Input: part model. Units: mm. Frame: model coordinates. A direction names the side the tool comes from. Coordinates: 2 decimals unless noted, no trailing zeros. Loops run counter-clockwise (first coordinate to the right, second up) from the corner with the lowest first, then second, coordinate; pieces in that order, holes last. Notation, with made-up numbers: (6, 2.5) - (26, 2.5) arc R12 cw to (26, 11.5) - close; hole circle Ø6 at (74, 28.25). An arc over 180 degrees is marked (long way). Write item = value, one per line. Start each with the question number.
from build123d import *

# Parameters (mm, degrees)
BOSS_EXTRUDE1_DEPTH = 2.54
SKETCH2_R           = 5.207
BOSS_EXTRUDE2_DEPTH = 12.7
SKETCH6_R           = 4
BOSS_EXTRUDE3_DEPTH = 5.08
FILLET1_R           = 0.508


with BuildPart() as part:
    # Sketch1 → Boss-Extrude1 (new body)
    with BuildSketch(Plane(origin=(0, 0, 0), x_dir=(1, 0, 0), z_dir=(0, 1, 0))):
        Polygon((10.998522628, 0), (5.499261314, 9.525), (-5.499261314, 9.525), (-10.998522628, 0), (-5.499261314, -9.525), (5.499261314, -9.525), align=None)
    extrude(amount=BOSS_EXTRUDE1_DEPTH)

    # Sketch2 → Boss-Extrude2 (add)
    with BuildSketch(Plane(origin=(0, 2.54, 0), x_dir=(1, 0, 0), z_dir=(0, 1, 0))):
        Circle(SKETCH2_R)
    extrude(amount=BOSS_EXTRUDE2_DEPTH)

    # Sketch6 → Boss-Extrude3 (add)
    with BuildSketch(Plane(origin=(0, 0, 0), x_dir=(-1, 0, 0), z_dir=(0, -1, 0))):
        Circle(SKETCH6_R)
    extrude(amount=BOSS_EXTRUDE3_DEPTH)

    # Fillet1
    fillet1_edges = [part.edges().sort_by_distance(p)[0] for p in [
        (0, 2.54, -9.525),
        (5.499261314, 1.27, 9.525),
        (-5.499261314, 1.27, 9.525),
        (-10.998522628, 1.27, 0),
        (-5.499261314, 1.27, -9.525),
        (5.499261314, 1.27, -9.525),
        (10.998522628, 1.27, 0),
        (-8.248891971, 2.54, -4.7625),
        (-8.248891971, 2.54, 4.7625),
        (0, 2.54, 9.525),
        (8.248891971, 2.54, 4.7625),
        (8.248891971, 2.54, -4.7625),
    ]]
    fillet(fillet1_edges, radius=FILLET1_R)


solid = part.part
Item 1: Access query for faces 1 (the flat face through (0, 1, -9.525)), 2 (the flat face through (4, 2.54, -4)), 3 (the cylindrical face through (0.867, -2.504, 3.905)). Directions: +Z, -Z, +X, -X, +Y, -Y. A direction counts if a zero-diameter tool reaches every point of the face in a straight line with its end or side. Return the directions, or none.
Item 2: Cut plane C-C on x = -4.75. Return loops of the section in (y, z) (3 decimals), plus the area to 3 significant figures.
Item 3: Cut plane D-D on y = -3. Return loops of the section in (x, z).
Item 4: Pin query (flat end, axial travel): pin 1 (10 mm diameter, centred on y = 10.5, z = -4.5, fed in from +X); pin 2 (3 mm diameter, centred on x = 0.5, y = -2, fed in from -Z); pin 3 (2 mm diameter, centred on x = -8.5, z = -2.5, fed in from -Y); pin 4 (2 mm diameter, centred on x = 7, y = -1.5, fed in from -Z). Return the tip coordinate at first contact, or that it passes through.
Item 5: Ray query, line 1 (Y direction, x = 2.5, z = -8.25); line 2 (X direction, y = 9.75, z = -3); line 3 (X direction, y = 3.75, z = 4.75). Return the intervals inside material, ascending.
Item 6: Cut plane B-B on y = 1.5. Return loops of the section in (x, z) (3 decimals), plus the area to 3 significant figures.
Item 7: Cut plane A-A on x = 0. Return loops of the section in (y, z) (3 decimals).
Recorded:
q1.face_1 = -Z, +X, -X, +Y, -Y
q1.face_2 = +Y
q1.face_3 = -Y
q2.outline = (0, -9.525) - (2.032, -9.525) arc R0.508 ccw to (2.54, -9.017) - (2.54, -2.133) - (15.24, -2.133) - (15.24, 2.133) - (2.54, 2.133) - (2.54, 9.017) arc R0.508 ccw to (2.032, 9.525) - (0, 9.525) - close
q2.area = 102 mm²
q3.outline = circle Ø8 at (0, 0)
q4.pin_1 = 5.21
q4.pin_2 = -4
q4.pin_3 = 0
q4.pin_4 = through
q5.line_1 = 0 to 2.54
q5.line_2 = -4.26 to 4.26
q5.line_3 = -2.13 to 2.13
q6.outline = (-10.852, -0.254) - (-5.646, -9.271) arc R0.508 ccw to (-5.206, -9.525) - (5.206, -9.525) arc R0.508 ccw to (5.646, -9.271) - (10.852, -0.254) arc R0.508 ccw to (10.852, 0.254) - (5.646, 9.271) arc R0.508 ccw to (5.206, 9.525) - (-5.206, 9.525) arc R0.508 ccw to (-5.646, 9.271) - (-10.852, 0.254) arc R0.508 ccw to start
q6.area = 314 mm²
q7.outline = (-5.08, -4) - (0, -4) - (0, -9.525) - (2.032, -9.525) arc R0.508 ccw to (2.54, -9.017) - (2.54, -5.207) - (15.24, -5.207) - (15.24, 5.207) - (2.54, 5.207) - (2.54, 9.017) arc R0.508 ccw to (2.032, 9.525) - (0, 9.525) - (0, 4) - (-5.08, 4) - close
